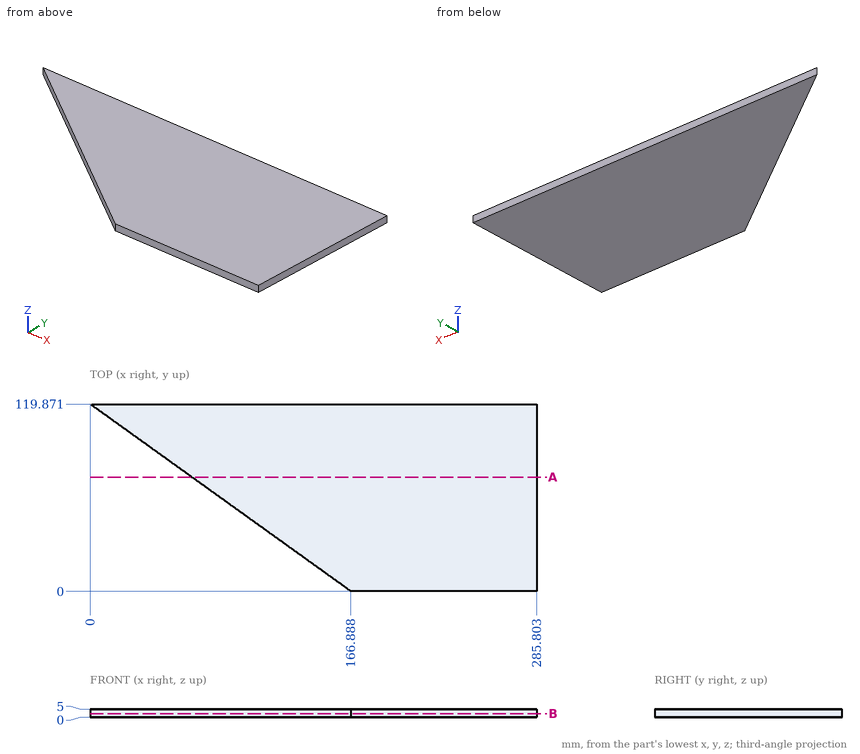
For this review, use the dimensioned drawing (mm, ordinates from the lowest corner) and the shaded views. Round coordinates to 2 decimals unless told otherwise and drop trailing zeros. Write each loop counter-clockwise with the first axis right and the second up, starting at its lowest first coordinate (ties: lowest second). Pieces come first, ordered by that corner, then holes. Notation, with made-up numbers: M 28.25,52 L 58.25,52 A15 ccw 58.25,61 Z; hole C 82.5,49 d9. An arc over 180 degrees is marked long. Write item = value, one per line. Start each with the question number.
(1) We need section A-A (y = 73). Give the boundary of the cut face in (x, z) (1 decimal).
(2) We need section B-B (z = 2.2). Give the boundary of the cut face in (x, y), then the cut area to 3 significant figures.
(3) For line 1 along X through (y, z) = (100.5, 2.45) (1 decimal); line 2 along Y through (x, z) = (124, 3.15) (1 decimal); line 3 along X through (y, z) = (83, 1.35) (1 decimal), list the stretches that pass through material, from the lowest coordinate up.
Results found:
q1.outline = M 65.3,0 L 285.8,0 L 285.8,5 L 65.3,5 Z
q2.outline = M 0,119.87 L 166.89,0 L 285.8,0 L 285.8,119.87 Z
q2.area = 24,300 mm²
q3.line_1 = 27 to 285.8
q3.line_2 = 30.8 to 119.9
q3.line_3 = 51.3 to 285.8
